The figure shows three views and two pictorial views of one solid part (mm, origin at its lowest corner). Answer the questions. A direction names the side the tool comes from. Give positions to 0.01 mm unless a question says otherwise; leave off trailing zeros. Loops run counter-clockwise (first coordinate to the right, second up) from the corner with the lowest first, then second, coordinate; pieces in that order, holes last. Notation, with made-up numbers: M 57,68 L 107,68 A22 cw 107,82 Z; hole C 68,40 d7. An arc over 180 degrees is marked long. Answer in a Markdown table with one row per item. Add a question column.
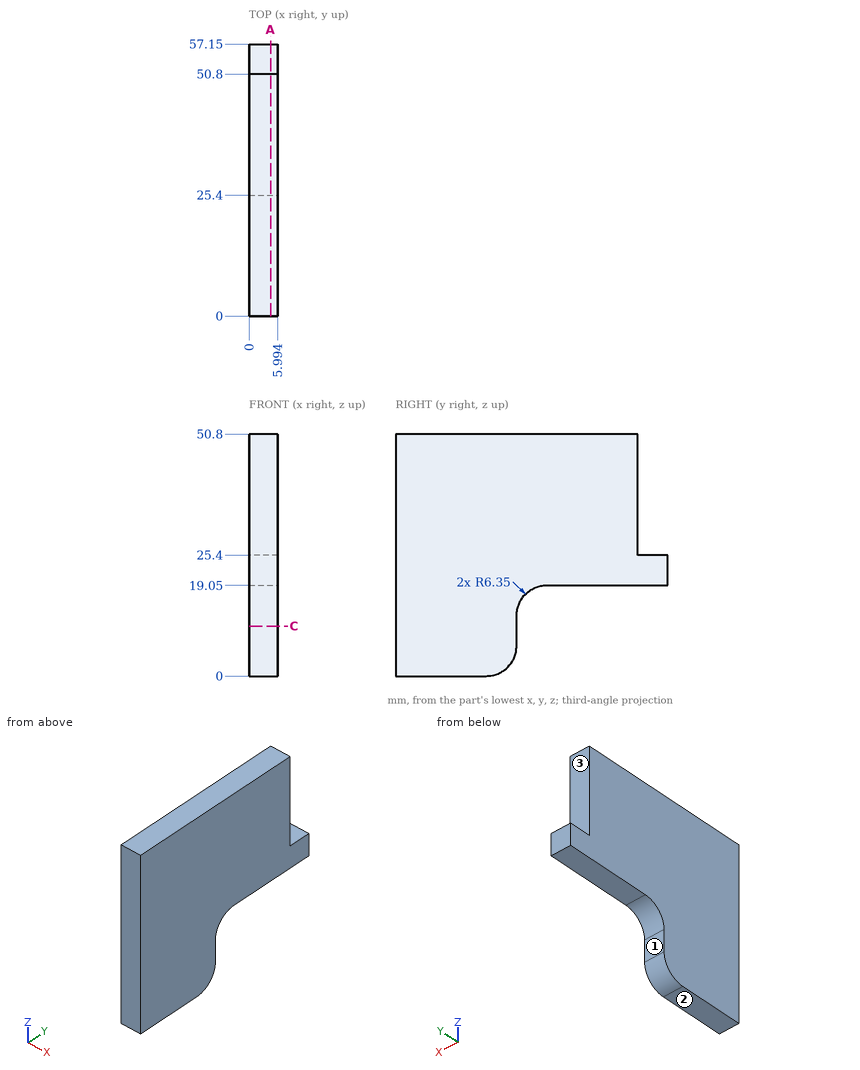
(1) Section A-A, the plane x = 4.5 is taken. Determine the outline of the cut face in (y, z).
(2) This flat-tipped pin is pushed along its axis until it touches: P1, Ø3, axis at x = 3, z = 11, coming from the +Y side. Where does it stop, or does it pass through?
(3) Section C-C, the plane z = 10.5 is taken. Determine the outline of the cut face in (x, y) (1 decimal).
(4) Which of the six approach directions +Z, -Z, +X, -X, +Y, -Y give full straight-line access (tool end or side, diameter ignored) to the marked faces 1, 2 and 3?
(5) Consider line 1 along Z through (x, y) = (0.35, 50.5); line 2 along Y through (x, z) = (2.8, 32); line 3 along Z through (x, y) = (0.9, 54). Determine where each line is inside the solid, lowest interval first. Write a range as from..to.
Numbers:
| question | item | result |
|---|---|---|
| 1 | outline | M 0,0 L 19.05,0 A6.35 ccw 25.4,6.35 L 25.4,12.7 A6.35 cw 31.75,19.05 L 57.15,19.05 L 57.15,25.4 L 50.8,25.4 L 50.8,50.8 L 0,50.8 Z |
| 2 | P1 | stops at y = 25.4 |
| 3 | outline | M 0,0 L 6,0 L 6,25.4 L 0,25.4 Z |
| 4 | face 1 | -Z, +X, -X, +Y |
| 4 | face 2 | -Z, +X, -X, +Y, -Y |
| 4 | face 3 | +Z, +X, -X, +Y |
| 5 | line 1 | z = 19.05..50.8 |
| 5 | line 2 | y = 0..50.8 |
| 5 | line 3 | z = 19.05..25.4 |
